CAD build for the part. Positions are in the model's coordinates, mm. Face numbers are marked on the shaded views. A direction names the side the tool comes from. Give positions to 0.01 mm unless a question says otherwise; leave off trailing zeros. Loops run counter-clockwise (first coordinate to the right, second up) from the corner with the lowest first, then second, coordinate; pieces in that order, holes last.
```python
from build123d import *

# Parameters (mm, degrees)
CUT_EXTRUDE1_DEPTH = 10
CUT_EXTRUDE2_DEPTH = 18
CIRPATTERN1_COUNT  = 3
CUT_EXTRUDE3_START = 21.741254
CUT_EXTRUDE3_DEPTH = 4


with BuildPart() as part:
    # Sketch1 → Revolve1 (revolve)
    with BuildSketch(Plane.XY, mode=Mode.PRIVATE) as revolve1_sk:
        Polygon((0, 2.5), (12.6, 2.5), (12.6, 3), (17.6, 3), (17.6, 5), (20.741253759, 5), (20.741253759, 2), (25.741253759, 2), (25.741253759, 0), (0, 0), align=None)
    revolve(revolve1_sk.sketch.rotate(Axis((0, 0, 0), (1, 0, 0)), 90), axis=Axis((0, 0, 0), (1, 0, 0)))

    # Sketch2 → Cut-Extrude1 (cut)
    with BuildSketch(Plane(origin=(0, 0, 0), x_dir=(0, 0, -1), z_dir=(1, 0, 0))):
        Polygon((0, 1.732050808), (-1.5, 0.866025404), (-1.5, -0.866025404), (0, -1.732050808), (1.5, -0.866025404), (1.5, 0.866025404), align=None)
    extrude(amount=CUT_EXTRUDE1_DEPTH, mode=Mode.SUBTRACT)

    # Sketch3 → Cut-Extrude2 (cut)
    with BuildSketch(Plane(origin=(0, 0, 0), x_dir=(1, 0, 0), z_dir=(0, 1, 0))):
        with BuildLine():
            Line((5.5, 1), (5.5, -1))
            ThreePointArc((5.5, -1), (5, -1.5), (4.5, -1))
            Line((4.5, -1), (4.5, 1))
            ThreePointArc((4.5, 1), (5, 1.5), (5.5, 1))
        make_face()
    cut_extrude2 = extrude(amount=CUT_EXTRUDE2_DEPTH, mode=Mode.SUBTRACT)

    # CirPattern1: Cut-Extrude2 ×3 about axis
    cirpattern1_axis = Axis((0, 0, 0), (-1, 0, 0))
    for i in range(1, CIRPATTERN1_COUNT):
        add(cut_extrude2.rotate(cirpattern1_axis, i * 360 / CIRPATTERN1_COUNT), mode=Mode.SUBTRACT)

    # Sketch4 → Cut-Extrude3 (cut)
    with BuildSketch(Plane(origin=(0, 0, 0), x_dir=(0, 0, -1), z_dir=(1, 0, 0)).offset(CUT_EXTRUDE3_START)):
        with BuildLine():
            Line((0.707106781, 0.25), (-0.707106781, 0.25))
            ThreePointArc((-0.707106781, 0.25), (-0.126826484, -0.73919892), (0.75, 0))
            ThreePointArc((0.75, 0), (0.73919892, 0.126826484), (0.707106781, 0.25))
        make_face()
    extrude(amount=CUT_EXTRUDE3_DEPTH, mode=Mode.SUBTRACT)


solid = part.part
```
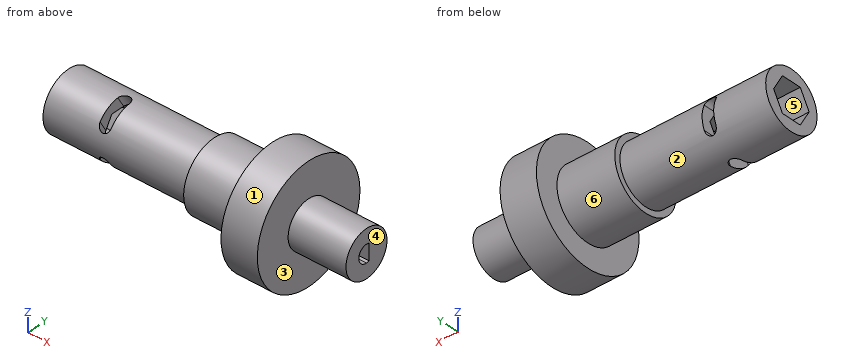
1. Pull direction Y, two halves, no side cores. Call the marked faces 4, 5 and 6: released by +Y, released by -Y, zero draft, split by the parting line, or undercut.
Responses:
face 4: zero draft
face 5: undercut
face 6: split by the parting line
2. Saw through at A-A, the plane x = 8.5. List the corners of the cut face in (y, z).
Responses:
outline: circle Ø5 at (0, 0); hole (-1.73, 0) - (-0.87, -1.5) - (0.87, -1.5) - (1.73, 0) - (0.87, 1.5) - (-0.87, 1.5) - close
3. Saw through at C-C, the plane x = 16.5. List the corners of the cut face in (y, z), and give its area (3 significant figures).
Responses:
outline: circle Ø6 at (0, 0)
area: 28.3 mm2
4. Drop flat-ended pins along their axis: pin 1 (4 mm diameter, centred on x = 4.5, z = -2, fed in from +Y); pin 2 (0.9 mm diameter, centred on y = 0, z = 0, fed in from -X); pin 3 (1.5 mm diameter, centred on y = 1, z = -3, fed in from -X); pin 4 (0.9 mm diameter, centred on x = 3.5, y = 0.5, fed in from -Z). Give the stop position or say it passes through.
Responses:
pin 1: stops at y = 2.5
pin 2: stops at x = 10
pin 3: stops at x = 0
pin 4: stops at z = -2.5
5. Probe line 1 along Y through (x, z) = (22.6, 0); line 2 along X through (y, z) = (0.5, 0.75); line 3 along X through (y, z) = (-1, 2.75). List the from-to ranges inside material, lowest first.
Responses:
line 1: y = -2 to -0.75, 0.25 to 2
line 2: x = 10 to 25.74
line 3: x = 12.6 to 20.74
6. Tool access for the marked faces 1, 2 and 3: list every direction of +Z, -Z, +X, -X, +Y, -Y with a clear straight run to the whole face (end or side of a thin tool).
Responses:
face 1: +X, -X
face 2: -X
face 3: +X
7. Saw through at D-D, the plane z = 3.5. List the corners of the cut face in (x, y), and give its area (3 significant figures).
Responses:
outline: (17.6, -3.57) - (20.74, -3.57) - (20.74, 3.57) - (17.6, 3.57) - close
area: 22.4 mm2
8. Saw through at B-B, the plane y = -3.25. List the corners of the cut face in (x, z), and give its area (3 significant figures).
Responses:
outline: (17.6, -3.8) - (20.74, -3.8) - (20.74, 3.8) - (17.6, 3.8) - close
area: 23.9 mm2
